The listing builds one solid part. Answer for the finished solid, in the listing's coordinates (mm). Face numbers are marked on the shaded views. Coordinates: 2 decimals unless noted, no trailing zeros. Loops run counter-clockwise (first coordinate to the right, second up) from the corner with the lowest first, then second, coordinate; pieces in that order, holes last. Notation, with made-up numbers: M 74.25,61 L 113.25,61 A24 ccw 113.25,93 Z; hole C 14,3 d1. An arc over 180 degrees is marked long. Answer in a Markdown table with one row per item. Add a question column.
from build123d import *

# Parameters (mm, degrees)
FILLET1_R = 0.508
FILLET2_R = 1.524


with BuildPart() as part:
    # Sketch1 → Revolve1 (revolve)
    with BuildSketch(Plane(origin=(0, 0, 0), x_dir=(0, 0, -1), z_dir=(1, 0, 0)), mode=Mode.PRIVATE) as revolve1_sk:
        with BuildLine():
            Line((-10.7442, 22.410197806), (-10.7442, 0))
            Line((-10.7442, 0), (-13.9192, 0))
            Line((-13.9192, 0), (-13.9192, 24.13))
            add(Edge.make_bspline(
                [(-13.9192, 24.13), (-10.066559664, 27.411628122), (-4.86398701, 28.085571939), (0, 27.94)],
                knots=[0, 0, 0, 0, 1, 1, 1, 1], degree=3))
            Line((0, 27.94), (0, 25.475077416))
            add(Edge.make_bspline(
                [(-10.343014188, 23.11581757), (-7.133322616, 24.732985356), (-3.68565122, 25.519405304), (0, 25.475077416)],
                knots=[0.040116886, 0.040116886, 0.040116886, 0.040116886, 1, 1, 1, 1], degree=3))
            Line((-10.343014188, 23.11581757), (-10.343014188, 22.410197806))
            Line((-10.343014188, 22.410197806), (-10.7442, 22.410197806))
        make_face()
    revolve(revolve1_sk.sketch.rotate(Axis((0, 0, 0), (0, 1, 0)), 180), axis=Axis((0, 0, 0), (0, 1, 0)))

    # Fillet1
    fillet1_edges = [part.edges().sort_by_distance(p)[0] for p in [
        (0, 0, 10.7442),
    ]]
    fillet(fillet1_edges, radius=FILLET1_R)

    # Fillet2
    fillet2_edges = [part.edges().sort_by_distance(p)[0] for p in [
        (0, 24.13, 13.9192),
    ]]
    fillet(fillet2_edges, radius=FILLET2_R)


solid = part.part
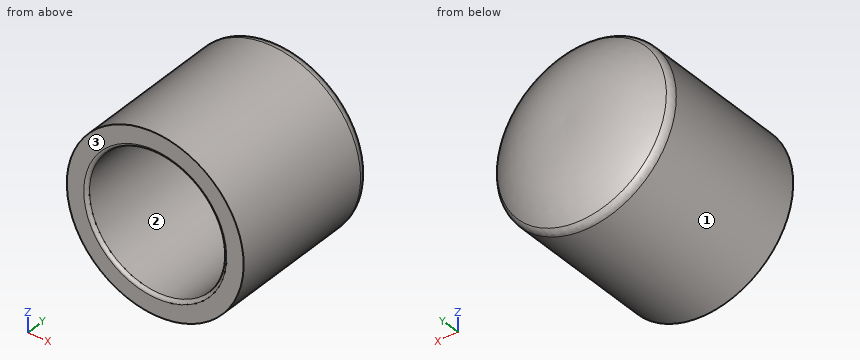
(1) The mould has two halves that part along Z. Classify the marked faces 1, 2 and 3: released by +Z, released by -Z, zero draft, split by the parting line, or undercut.
(2) Each of these flat-tipped pins is pushed along its axis until it touches: pin 1 (10 mm diameter, centred on x = 10, z = 7, fed in from +Y); pin 2 (1 mm diameter, centred on x = -1, y = 21.5, fed in from +Z); pin 3 (1.5 mm diameter, centred on x = 10.5, z = 4, fed in from +Y). Where does it stop, or does it pass through?
(3) Straight lines are drawn through the part: line 1 (X direction, y = 7.5, z = 0); line 2 (X direction, y = 22.6, z = 0); line 3 (Z direction, x = 9.5, y = 3.75). For each, find the intervals that lie inside material, in ascending order.
(4) A cutting plane is placed at A-A (y = 18.5). Give the vertices of the cut face in (x, z).
Solved:
| question | item | result |
|---|---|---|
| 1 | face 1 | split by the parting line |
| 1 | face 2 | undercut |
| 1 | face 3 | zero draft |
| 2 | pin 1 | stops at y = 27.35 |
| 2 | pin 2 | stops at z = 13.91 |
| 2 | pin 3 | stops at y = 26.28 |
| 3 | line 1 | x = -13.92 to -10.74, 10.74 to 13.92 |
| 3 | line 2 | x = -13.92 to -10.34, 10.34 to 13.92 |
| 3 | line 3 | z = -10.17 to -5.02, 5.02 to 10.17 |
| 4 | outline | C 0,0 d27.84; hole C 0,0 d21.49 |
